For this review, take the finished solid that the model builds, in its own axes (mm). A direction names the side the tool comes from. Round coordinates to 2 decimals unless told otherwise and drop trailing zeros. Order: outer loops, then holes, each group sorted by start corner. A loop starts at its lowest first (then second) coordinate and runs counter-clockwise, first axis right, second up. Notation, with made-up numbers: M 28,49.25 L 70,49.25 A32 cw 70,76.25 Z; hole C -20,-27.5 d3. An arc over 180 degrees is marked long. Answer as a JSON object with one key per item and string values.
Autodesk Inventor part; units mm, degrees
ref_plane "YZ Plane" through (0, 0, 0) normal (1, 0, 0) x (0, 1, 0)
ref_plane "XZ Plane" through (0, 0, 0) normal (0, 1, 0) x (-1, 0, 0)
ref_plane "XY Plane" through (0, 0, 0) normal (0, 0, 1) x (1, 0, 0)
sketch "Sketch1" plane through (0, 0, 0) normal (0, 1, 0) x (-1, 0, 0)
  circle A0 centre (0, 0) radius 25
  circle A1 centre (0, 0) radius 25.9
  circle A2 centre (0, 0) radius 26.8
  dimension "d0" = 50
  dimension "d1" = 51.8
  dimension "d2" = 53.6
extrude "Extrusion1" add sketch "Sketch1" along normal blind 75 and the other way blind 80 contours A1
extrude "Extrusion2" add sketch "Sketch1" along normal blind 75 and the other way blind 75 contours A2
sketch "Sketch4" plane through (0, 0, 0) normal (0, 0, 1) x (1, 0, 0)
  line L0 (65, 99.9302) -> (65, 38.564)
  line L1 (65, 38.564) -> (25, 5)
  line L2 (25, 5) -> (25, 75)
  line L3 (25, 75) -> (65, 88.564)
  line L4 (65, 88.564) -> (65, 99.9302)
  line L5 (-25, 75) -> (25, 75)
  line L6 (-25, 75) -> (25, 75)
  line L7 (25.9, -80) -> (25, -80)
  line L8 (25, -80) -> (25, 75)
  line L9 (26.8, 75) -> (26.8, -75)
  line L10 (-25, -80) -> (-25.9, -80)
  line L11 (-26.8, -75) -> (-26.8, 75)
  line L12 (-25, 75) -> (-25, -80)
  line L13 (25, 75) -> (26.8, 75)
  line L14 (-26.8, 75) -> (-25, 75)
  line L15 (26.8, -75) -> (25.9, -75)
  line L16 (25.9, -75) -> (25.9, -80)
  line L17 (-25.9, -80) -> (-25.9, -75)
  line L18 (-25.9, -75) -> (-26.8, -75)
  point P0 (0, 0)
  point P1 (26.8, 96)
  point P2 (-26.8, 96)
  point P3 (26.8, 6.5104)
  point P4 (15.9, -100)
  point P5 (-15.9, -100)
  point P6 (25, 5)
  dimension "d18" = 70
  dimension "d21" = 50
  dimension "d24" = 50
  dimension "d25" = 40
extrude "Extrusion4" add sketch "Sketch4" along normal mid plane 3.6 contours L0 L1 L9 L13 L3 | L13 L9 L1 L2 | L9 L15 L16 L7 L8 L1
pattern_circular "Circular Pattern2" count 3 over 360 about axis through (0, -10, 0) along (0, 1, 0) of "Extrusion4"
properties part number "tail" material "ABS Plastic"
1) Insertion check: P1, Ø6, axis at x = 47, z = -5, coming from the +Y side; P2, Ø3, axis at y = -77.5, z = 0, coming from the +X side; P3, Ø1.1, axis at y = -25, z = -0.5, coming from the +X side; P4, Ø8, axis at x = 18.5, y = -50, coming from the -Z side. Each pin has a flat end and moves straight along its axis. Give the tip position at first contact, or say it passes through.
Geometry check:
{"P1": "passes through", "P2": "stops at x = 25.9", "P3": "stops at x = 26.8", "P4": "stops at z = -22.54"}
2) Machinability: for faces 1 (the flat face through (14, -75, 22)), 2 (the flat face through (25.9, -77, 0)), 3 (the flat face through (-25.4, 75, 0.1)), 4 (the cylindrical face through (13.26, -77.46, -22.25)), which of the approach directions +Z, -Z, +X, -X, +Y, -Y give a long, thin tool a straight path to every point of the face, cutting with its end or side? Answer none if there is none.
Geometry check:
{"face 1": "-Y", "face 2": "+Z, -Z, +X, -Y", "face 3": "-X, +Y", "face 4": "-Z, -Y"}
3) Add section D-D on y = 20. State the section outline as (x, z) points, and give its area (3 significant figures).
Geometry check:
{"outline": "M -23,-36.23 L -19.88,-38.03 L -11.81,-24.06 A26.8 ccw 26.74,-1.8 L 42.88,-1.8 L 42.88,1.8 L 26.74,1.8 A26.8 ccw -11.81,24.06 L -19.88,38.03 L -23,36.23 L -14.93,22.26 A26.8 ccw -14.93,-22.26 Z; hole C 0,0 d50", "area": "467 mm²"}
4) Add section C-C on y = -33.5. State the section outline as (x, z) points.
Geometry check:
{"outline": "M -14.96,-22.31 L -11.84,-24.11 L -11.81,-24.06 A26.8 ccw 26.74,-1.8 L 26.8,-1.8 L 26.8,1.8 L 26.74,1.8 A26.8 ccw -11.81,24.06 L -11.84,24.11 L -14.96,22.31 L -14.93,22.26 A26.8 ccw -14.93,-22.26 Z; hole C 0,0 d50"}
5) Add section A-A on x = 0. State the section outline as (y, z) points.
Geometry check:
{"outline": "M -80,-25.9 L -75,-25.9 L -75,-26.8 L 75,-26.8 L 75,-25 L -80,-25 Z; M -80,25 L 75,25 L 75,26.8 L -75,26.8 L -75,25.9 L -80,25.9 Z"}
6) For L1, parallel to X at y = -16, z = 0; L2, parallel to X at y = 44.5, z = 0; L3, parallel to Z at x = -7.5, y = -13.5, list the stretches that pass through material, from the lowest coordinate up.
Geometry check:
{"L1": "x = -26.8 to -25, 25 to 26.8", "L2": "x = -26.8 to -25, 25 to 65", "L3": "z = -25.73 to -23.85, 23.85 to 25.73"}
7) Add section B-B on z = -17.5. State the section outline as (x, y) points.
Geometry check:
{"outline": "M -20.3,-75 L -19.09,-75 L -19.09,-80 L -17.85,-80 L -17.85,75 L -20.3,75 Z; M 17.85,-80 L 19.09,-80 L 19.09,-75 L 20.3,-75 L 20.3,75 L 17.85,75 Z"}
